```python
from build123d import *

# Parameters (mm, degrees)
SKETCH1_R           = 3.95
BOSS_EXTRUDE1_DEPTH = 6
SKETCH2_R           = 6
BOSS_EXTRUDE2_DEPTH = 1
SKETCH3_W           = 24
SKETCH3_H           = 14
SKETCH3_H_2         = 26
SKETCH3_R           = 6
BOSS_EXTRUDE3_DEPTH = 21
SKETCH6_W           = 64
SKETCH6_H           = 2
BOSS_EXTRUDE5_DEPTH = 21
SKETCH8_W           = 20
SKETCH8_H           = 20
SKETCH8_H_2         = 6
CUT_EXTRUDE1_DEPTH  = 49.020828814
SKETCH9_W           = 4.63141447
SKETCH9_H           = 1.5
CUT_EXTRUDE2_DEPTH  = 6
BOSS_EXTRUDE6_DEPTH = 1
SKETCH11_W          = 20
SKETCH11_H          = 20
CUT_EXTRUDE3_DEPTH  = 52.46843693


with BuildPart() as part:
    # Sketch1 → Boss-Extrude1 (new body)
    with BuildSketch(Plane(origin=(0, 0, 0), x_dir=(1, 0, 0), z_dir=(0, 1, 0))):
        with Locations(Location((0, 0, 0), (0, 0, 270))):
            Circle(SKETCH1_R)
    extrude(amount=BOSS_EXTRUDE1_DEPTH)

    # Sketch2 → Boss-Extrude2 (add)
    with BuildSketch(Plane.XZ):
        with Locations(Location((0, 0, 0), (0, 0, 270))):
            Circle(SKETCH2_R)
    extrude(amount=BOSS_EXTRUDE2_DEPTH)

    # Sketch3 → Boss-Extrude3 (add)
    # profile 1 of 3: a face of its own
    with BuildSketch(Plane.XZ.offset(1)):
        with Locations((0, 20)):
            Rectangle(SKETCH3_W, SKETCH3_H)
    # profile 2 of 3: a face of its own
    with BuildSketch(Plane.XZ.offset(1)):
        Rectangle(SKETCH3_W, SKETCH3_H_2)
        with Locations(Location((0, 0, 0), (0, 0, 270))):
            Circle(SKETCH3_R, mode=Mode.SUBTRACT)
    # profile 3 of 3: a face of its own
    with BuildSketch(Plane.XZ.offset(1)):
        with Locations(Location((0, 0, 0), (0, 0, 270))):
            Circle(SKETCH3_R)
    extrude(amount=BOSS_EXTRUDE3_DEPTH)

    # Sketch6 → Boss-Extrude5 (add)
    with BuildSketch(Plane.XZ.offset(22)):
        with Locations((0, 28)):
            Rectangle(SKETCH6_W, SKETCH6_H)
    extrude(amount=-BOSS_EXTRUDE5_DEPTH)

    # Sketch8 → Cut-Extrude1 (cut, through all)
    with BuildSketch(Plane(origin=(0, -1, 0), x_dir=(1, 0, 0), z_dir=(0, 1, 0))):
        with Locations((0, -17)):
            Rectangle(SKETCH8_W, SKETCH8_H)
        with Locations((0, 10)):
            Rectangle(SKETCH8_W, SKETCH8_H_2)
    extrude(amount=-CUT_EXTRUDE1_DEPTH, mode=Mode.SUBTRACT)

    # Sketch9 → Cut-Extrude2 (cut)
    with BuildSketch(Plane(origin=(0, 6, 0), x_dir=(1, 0, 0), z_dir=(0, 1, 0))):
        with Locations((0, -3.95)):
            Rectangle(SKETCH9_W, SKETCH9_H)
    extrude(amount=-CUT_EXTRUDE2_DEPTH, mode=Mode.SUBTRACT)

    # Sketch10 → Boss-Extrude6 (add)
    with BuildSketch(Plane.XZ.offset(22)):
        Polygon((-32, 29), (32, 29), (32, 27), (12, -13), (-12, -13), (-32, 27), align=None)
    extrude(amount=BOSS_EXTRUDE6_DEPTH)

    # Sketch11 → Cut-Extrude3 (cut, through all)
    with BuildSketch(Plane(origin=(0, -22, 0), x_dir=(1, 0, 0), z_dir=(0, 1, 0))):
        with Locations((0, -17)):
            Rectangle(SKETCH11_W, SKETCH11_H)
    extrude(amount=-CUT_EXTRUDE3_DEPTH, mode=Mode.SUBTRACT)


solid = part.part
```
Geometry: final body of the model. Coordinates: model frame, mm. A direction names the side the tool comes from. Coordinates: 2 decimals unless noted, no trailing zeros. Order: outer loops, then holes, each group sorted by start corner. A loop starts at its lowest first (then second) coordinate and runs counter-clockwise, first axis right, second up. Notation, with made-up numbers: M 38.5,-3.5 L 45.5,-3.5 A24 cw 45.5,10.5 Z; hole C 84,66 d5. An arc over 180 degrees is marked long. Answer in a Markdown table with one row per item. Add a question column.
Q1. Section query D-D on z = 22.5. Return the cut outline in (x, y), and give its area (4 significant figures).
Q2. Line query: L1, parallel to X at y = -8.5, z = 20.5; L2, parallel to Z at x = 2.5, y = -3.5; L3, parallel to Y at x = -3.5, z = -10.5. Output: solid intervals per line, ascending.
Q3. Reachability of faces 1 (the flat face through (22, -12, 27)), 2 (the flat face through (-1, 0, -4)), 3 (the flat face through (0, -11, -7)) from +Z, -Z, +X, -X, +Y, -Y: full face, straight path, thin tool, end or side. Return the list, or none.
Q4. Section query A-A on z = 10. Return the cut outline in (x, y).
Q5. Contact query for flat-ended pins moving along their axis: P1, Ø4, axis at y = -10, z = -7.5, coming from the +X side; P2, Ø1.5, axis at x = 7, y = -9, coming from the -Z side; P3, Ø16, axis at x = -21, y = -6.5, coming from the -Z side; P4, Ø16, axis at y = -9.5, z = 20, coming from the -X side. Output: stop coordinate, or through.
Q6. Section query C-C on x = 0. Return the cut outline in (y, z).
Q7. Mould query, pull axis X, two halves, no side actions, for faces 4 (the flat face through (-10, -12, 17)), 5 (the flat face through (-22, -12, 27)), 6 (the flat face through (-32, -12, 28)). Classes: released by +X, released by -X, zero draft, split by the parting line, or undercut.
Q8. Section query B-B on y = -18.5. Return the cut outline in (x, z).
Completed:
| question | item | result |
|---|---|---|
| 1 | outline | M -29.75,-23 L -10,-23 L -10,-1 L -12,-1 L -12,-22 L -29.75,-22 Z; M 10,-23 L 29.75,-23 L 29.75,-22 L 12,-22 L 12,-1 L 10,-1 Z |
| 1 | area | 123.5 mm2 |
| 2 | L1 | x = -12 to -10, 10 to 12 |
| 2 | L2 | z = -7 to 7, 27 to 29 |
| 2 | L3 | y = -23 to -22 |
| 3 | face 1 | -Z, +X, +Y |
| 3 | face 2 | +Y |
| 3 | face 3 | -Z, +Y |
| 4 | outline | M -23.5,-23 L -10,-23 L -10,-1 L -12,-1 L -12,-22 L -23.5,-22 Z; M 10,-23 L 23.5,-23 L 23.5,-22 L 12,-22 L 12,-1 L 10,-1 Z |
| 5 | P1 | stops at x = 12 |
| 5 | P2 | stops at z = -7 |
| 5 | P3 | stops at z = 27 |
| 5 | P4 | stops at x = -32 |
| 6 | outline | M -23,-13 L -22,-13 L -22,-7 L -1,-7 L -1,-6 L 0,-6 L 0,-3.95 L 6,-3.95 L 6,3.2 L 0,3.2 L 0,6 L -1,6 L -1,7 L -23,7 Z; M -23,27 L -1,27 L -1,29 L -23,29 Z |
| 7 | face 4 | undercut |
| 7 | face 5 | zero draft |
| 7 | face 6 | released by -X |
| 8 | outline | M -32,27 L -12,27 L -12,-13 L -10,-13 L -10,-7 L 10,-7 L 10,-13 L 12,-13 L 12,27 L 32,27 L 32,29 L -32,29 Z; hole M -10,7 L 10,7 L 10,27 L -10,27 Z |
